Input: dimensioned drawing with shaded views. Units: mm. Origin: part minimum x, y, z. Round coordinates to 2 decimals unless told otherwise and drop trailing zeros. Loops run counter-clockwise (first coordinate to the right, second up) from the corner with the lowest first, then second, coordinate; pieces in that order, holes last. Notation, with made-up numbers: (85.5, 21) - (108.5, 21) arc R21 ccw to (108.5, 57) - close; hole circle Ø3 at (12.25, 30). An arc over 180 degrees is marked (long way). Write each question's results on one line, items separated by ' | '.
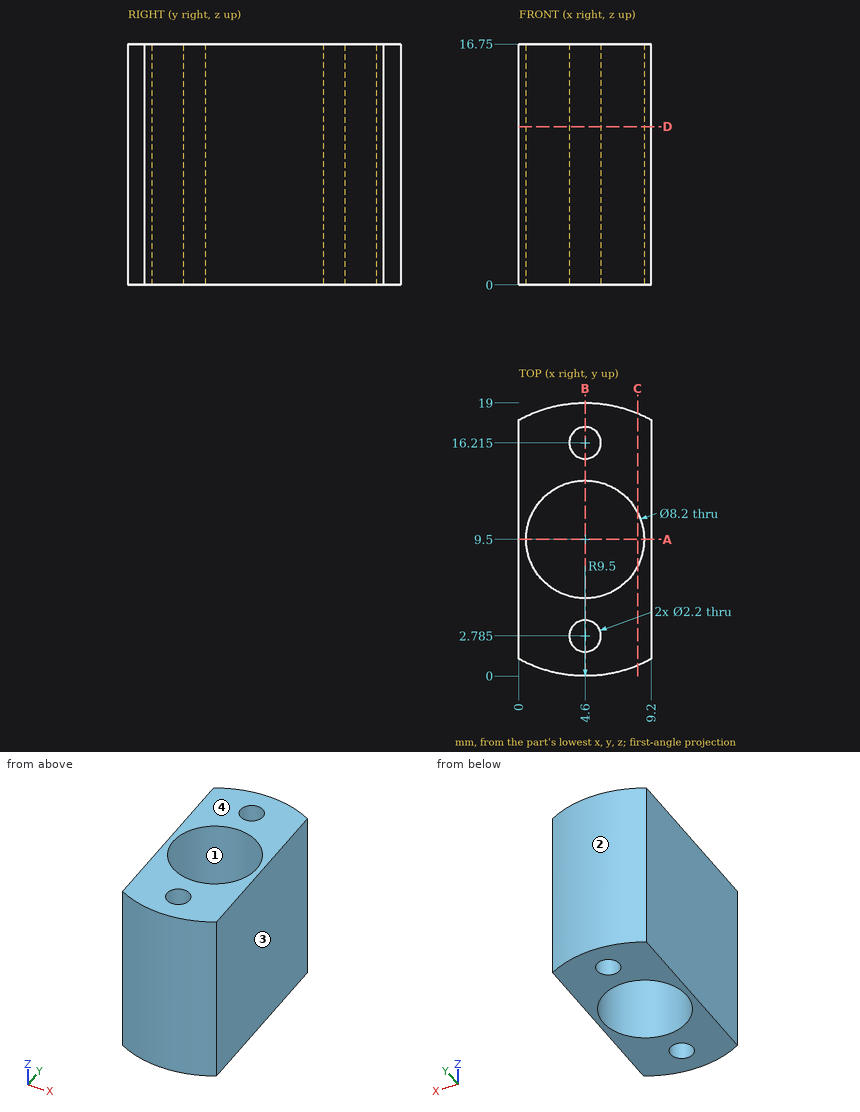
1. Section query B-B, the plane x = 4.6. Output: boundary loops of the cut face in (y, z) (3 decimals).
Answer:
outline: (0, 0) - (1.685, 0) - (1.685, 16.75) - (0, 16.75) - close; (3.885, 0) - (5.4, 0) - (5.4, 16.75) - (3.885, 16.75) - close; (13.6, 0) - (15.115, 0) - (15.115, 16.75) - (13.6, 16.75) - close; (17.315, 0) - (19, 0) - (19, 16.75) - (17.315, 16.75) - close
2. Section query C-C, the plane x = 8.25. Output: boundary loops of the cut face in (y, z), plus the area to 3 significant figures.
Answer:
outline: (0.73, 0) - (7.63, 0) - (7.63, 16.75) - (0.73, 16.75) - close; (11.37, 0) - (18.27, 0) - (18.27, 16.75) - (11.37, 16.75) - close | area: 231 mm^2
3. Line query: line 1 (Y direction, x = 5, z = 8.75); line 2 (Y direction, x = 6, z = 13.75); line 3 (Y direction, x = 7.5, z = 1.75). Output: solid intervals per line, ascending. Write a range as [from, to].
Answer:
line 1: [0.01, 1.76], [3.81, 5.42], [13.58, 15.19], [17.24, 18.99] | line 2: [0.1, 5.65], [13.35, 18.9] | line 3: [0.45, 6.6], [12.4, 18.55]
4. Contact query for a flat-ended pin moving along its axis: pin 1 (1.8 mm diameter, centred on x = 4.6, y = 16.215, fed in from -Z). Output: stop coordinate, or through.
Answer:
pin 1: through
5. Section query D-D, the plane z = 11. Output: boundary loops of the cut face in (x, y) (3 decimals).
Answer:
outline: (0, 1.188) arc R9.5 ccw to (9.2, 1.188) - (9.2, 17.812) arc R9.5 ccw to (0, 17.812) - close; hole circle Ø8.2 at (4.6, 9.5); hole circle Ø2.2 at (4.6, 2.785); hole circle Ø2.2 at (4.6, 16.215)
6. Mould query, pull axis X, two halves, no side actions, for the marked faces 1, 2, 3 and 4. Classes: pulls with the +X half, pulls with the -X half, needs draft (parallel to the pull), parting line crosses it, or undercut.
Answer:
face 1: undercut | face 2: parting line crosses it | face 3: pulls with the +X half | face 4: needs draft
7. Section query A-A, the plane y = 9.5. Output: boundary loops of the cut face in (x, z), plus the area to 4 significant figures.
Answer:
outline: (0, 0) - (0.5, 0) - (0.5, 16.75) - (0, 16.75) - close; (8.7, 0) - (9.2, 0) - (9.2, 16.75) - (8.7, 16.75) - close | area: 16.75 mm^2
